from build123d import *

# Parameters (mm, degrees)
SKETCH1_W            = 28
SKETCH1_H            = 24
BOSS_EXTRUDE1_DEPTH  = 4
SKETCH3_W            = 5
SKETCH3_H            = 24
BOSS_EXTRUDE2_DEPTH  = 30
LPATTERN1_COUNT      = 2
LPATTERN1_PITCH      = 34
M6_CLEARANCE_HOLE1_D = 6.6
CUT_EXTRUDE1_REACH   = 52.16
SKETCH8_R            = 3
SKETCH8_R_2          = 1.2
CIRPATTERN1_COUNT    = 4


with BuildPart() as part:
    # Sketch1 → Boss-Extrude1 (new body)
    with BuildSketch(Plane.XY):
        with Locations((14, 12)):
            Rectangle(SKETCH1_W, SKETCH1_H)
    boss_extrude1 = extrude(amount=BOSS_EXTRUDE1_DEPTH)

    # Sketch3 → Boss-Extrude2 (add)
    with BuildSketch(Plane(origin=(0, 0, 0), x_dir=(-1, 0, 0), z_dir=(0, 0, -1))):
        with Locations((-25.5, 12)):
            Rectangle(SKETCH3_W, SKETCH3_H)
    extrude(amount=BOSS_EXTRUDE2_DEPTH)

    # LPattern1: Boss-Extrude1 ×2
    with Locations(*[(0, 0, -i * LPATTERN1_PITCH) for i in range(1, LPATTERN1_COUNT)]):
        add(boss_extrude1)

    # M6 Clearance Hole1 (through all)
    with Locations(Plane.XY.offset(4)):
        with Locations((8, 12)):
            Hole(M6_CLEARANCE_HOLE1_D / 2)

    # Sketch8 → Cut-Extrude1 (cut, up to next)
    with BuildSketch(Plane(origin=(28, 0, 0), x_dir=(0, 0, -1), z_dir=(1, 0, 0)), mode=Mode.PRIVATE) as cut_extrude1_sk1:
        with Locations((15, 12)):
            Circle(SKETCH8_R)
    cut_extrude1_tool1 = extrude(cut_extrude1_sk1.sketch, amount=-CUT_EXTRUDE1_REACH, mode=Mode.PRIVATE) & part.part
    # Sketch8 → Cut-Extrude1 (cut, up to next)
    with BuildSketch(Plane(origin=(28, 0, 0), x_dir=(0, 0, -1), z_dir=(1, 0, 0)), mode=Mode.PRIVATE) as cut_extrude1_sk2:
        with Locations((8, 12)):
            Circle(SKETCH8_R_2)
    cut_extrude1_tool2 = extrude(cut_extrude1_sk2.sketch, amount=-CUT_EXTRUDE1_REACH, mode=Mode.PRIVATE) & part.part
    cut_extrude1_1 = cut_extrude1_tool1.solids().sort_by_distance((28, 12, -15))[0]
    add(cut_extrude1_1, mode=Mode.SUBTRACT)
    cut_extrude1_2 = cut_extrude1_tool2.solids().sort_by_distance((28, 12, -8))[0]
    add(cut_extrude1_2, mode=Mode.SUBTRACT)
    cut_extrude1 = cut_extrude1_1 + cut_extrude1_2  # Cut-Extrude1 as one shape, for the pattern or mirror that repeats it

    # CirPattern1: Cut-Extrude1 ×4 about axis
    cirpattern1_axis = Axis((0, 12, -15), (1, 0, 0))
    for i in range(1, CIRPATTERN1_COUNT):
        add(cut_extrude1.rotate(cirpattern1_axis, i * 360 / CIRPATTERN1_COUNT), mode=Mode.SUBTRACT)


solid = part.part
Work out the finished part from the listing and answer in its coordinate system (mm). A direction names the side the tool comes from. Give positions to 0.01 mm unless a question says otherwise; leave off trailing zeros. Order: outer loops, then holes, each group sorted by start corner. A loop starts at its lowest first (then second) coordinate and runs counter-clockwise, first axis right, second up. Notation, with made-up numbers: (-1, 1.25) -> (22, 1.25) arc R24 ccw to (22, 29.25) -> close; hole circle Ø8 at (52, 58.5). An arc over 180 degrees is marked (long way). Answer as a JSON object with one key per item and string values. Group by question number.
1. Flat-ended cylindrical pins translate along their axes: pin 1 Ø4 at (y, z) = (5, -15) entering from -X; pin 2 Ø10.5 at (x, y) = (8, 12) entering from -Z. Find the tip coordinate at first contact, or state that the pin passes through.
2. The mould has two halves that part along Y. Classify faces 3 (the flat face through (26, 0, -15)), 4 (the flat face through (26, 24, -15)), 5 (the cylindrical face through (25.5, 10.2, -12.6)), 6 (the flat face through (28, 12, -19)): released by +Y, released by -Y, zero draft, split by the parting line, or undercut.
3. Section D-D on z = -8 is taken. Determine the outline of the cut face in (x, y).
4. Section C-C on x = 4 is taken. Determine the outline of the cut face in (y, z).
5. Section A-A on z = -15 is taken. Determine the outline of the cut face in (x, y), plus the area to 3 significant figures.
6. A tool of negligible diameter and unlimited length cuts with its end or side. For faces 1 (the cylindrical face through (25.54, 10.83, -7.74)), 2 (the flat face through (23, 12, -11)), from which of +Z, -Z, +X, -X, +Y, -Y can it reach the whole face along a straight path? Write none if from no direction.
7. Consider line 1 along Z through (x, y) = (16, 3.5); line 2 along Y through (x, z) = (24.7, -22); line 3 along Y through (x, z) = (8, 1.1). Determine where each line is inside the solid, lowest interval first. Write a range as [from, to].
8. Section B-B on y = 5 is taken. Determine the outline of the cut face in (x, z).
Result sheet:
{
 "1": {"pin 1": "stops at x = 23", "pin 2": "stops at z = -34"},
 "2": {"face 3": "released by -Y", "face 4": "released by +Y", "face 5": "undercut", "face 6": "zero draft"},
 "3": {"outline": "(23, 0) -> (28, 0) -> (28, 10.8) -> (23, 10.8) -> close; (23, 13.2) -> (28, 13.2) -> (28, 24) -> (23, 24) -> close"},
 "4": {"outline": "(0, -34) -> (24, -34) -> (24, -30) -> (0, -30) -> close; (0, 0) -> (24, 0) -> (24, 4) -> (0, 4) -> close"},
 "5": {"outline": "(23, 0) -> (28, 0) -> (28, 3.8) -> (23, 3.8) -> close; (23, 6.2) -> (28, 6.2) -> (28, 9) -> (23, 9) -> close; (23, 15) -> (28, 15) -> (28, 17.8) -> (23, 17.8) -> close; (23, 20.2) -> (28, 20.2) -> (28, 24) -> (23, 24) -> close", "area": "66.0 mm^2"},
 "6": {"face 1": "+X, -X", "face 2": "-X, +Y, -Y"},
 "7": {"line 1": "z = [-34, -30], [0, 4]", "line 2": "y = [0, 10.8], [13.2, 24]", "line 3": "y = [0, 8.7], [15.3, 24]"},
 "8": {"outline": "(0, -34) -> (28, -34) -> (28, -16.2) -> (23, -16.2) -> (23, -30) -> (0, -30) -> close; (0, 0) -> (23, 0) -> (23, -13.8) -> (28, -13.8) -> (28, 4) -> (0, 4) -> close"}
}
